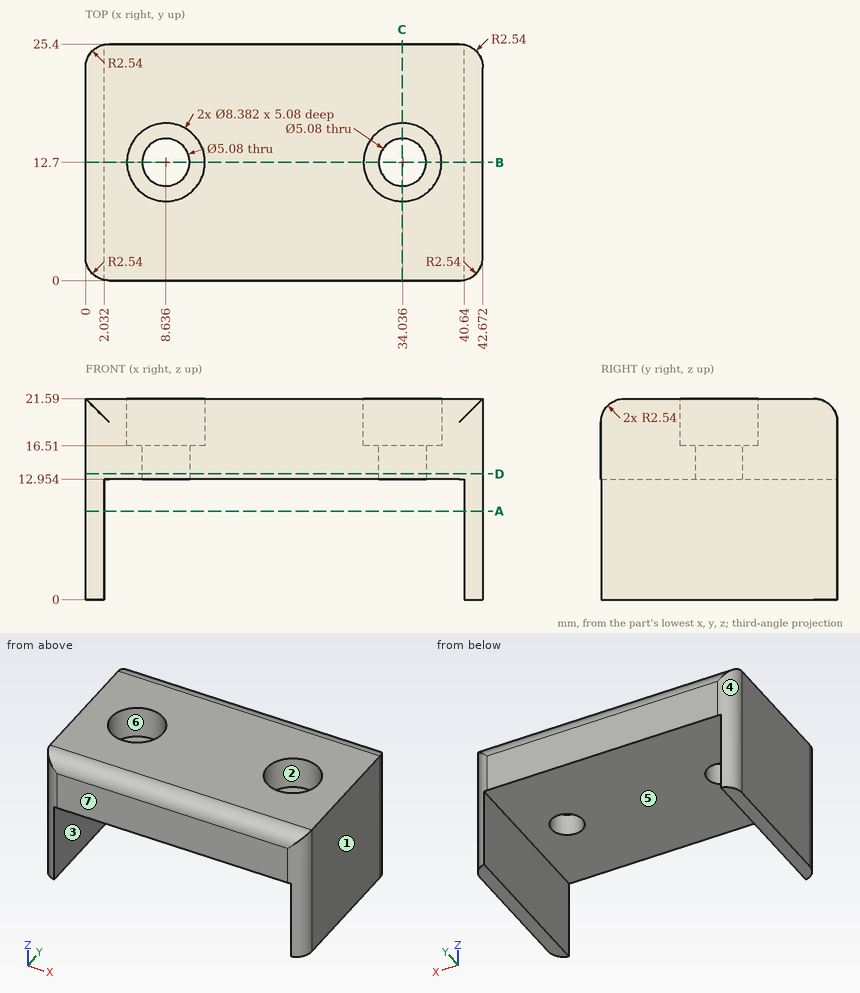
Here's the drawing with two shaded views (mm, measured from the low corner). I have some questions. A direction names the side the tool comes from. Give positions to 0.01 mm unless a question says otherwise; leave off trailing zeros. Loops run counter-clockwise (first coordinate to the right, second up) from the corner with the lowest first, then second, coordinate; pieces in that order, holes last. Notation, with made-up numbers: M 35,-10 L 88,-10 A20 ccw 88,14 Z; hole C 36.25,-25.75 d9. An arc over 180 degrees is marked long. One line per item, written item: value.
1) Imagine slicing it at B-B on y = 12.7. Write out the boundary of the cut face in (x, z) (3 decimals).
Geometry check:
outline: M 0,0 L 2.032,0 L 2.032,12.954 L 6.096,12.954 L 6.096,16.51 L 4.445,16.51 L 4.445,21.59 L 0,21.59 Z; M 11.176,12.954 L 31.496,12.954 L 31.496,16.51 L 29.845,16.51 L 29.845,21.59 L 12.827,21.59 L 12.827,16.51 L 11.176,16.51 Z; M 36.576,12.954 L 40.64,12.954 L 40.64,0 L 42.672,0 L 42.672,21.59 L 38.227,21.59 L 38.227,16.51 L 36.576,16.51 Z
2) On a 3-axis mill with a long thin cutter (end or side, diameter ignored), from which of +Z, -Z, +X, -X, +Y, -Y can I reach the whole of each face in a straight line? I mean the marked faces 5, 6 and 7. Say none if no direction works.
Geometry check:
face 5: -Z, +Y, -Y
face 6: +Z
face 7: +Z, -Z, +X, -X, -Y
3) Please list where these lines run through material, in increasing order: line 1 (X direction, y = 9.25, z = 7.25); line 2 (Z direction, x = 20.5, y = 3.75); line 3 (Z direction, x = 9.5, y = 10).
Geometry check:
line 1: x = 0 to 2.03, 40.64 to 42.67
line 2: z = 12.95 to 21.59
line 3: z = 12.95 to 16.51
4) I'm going to push flat-ended pins straight in: pin 1 (10 mm diameter, centred on y = 19.5, z = 7, fed in from -X); pin 2 (8 mm diameter, centred on x = 34.036, y = 12.7, fed in from +Z); pin 3 (10 mm diameter, centred on x = 19, y = 14.5, fed in from -Z); pin 4 (4.5 mm diameter, centred on x = 8.636, y = 12.7, fed in from +Z). Where does each tip first touch, or does it pass through?
Geometry check:
pin 1: stops at x = 0
pin 2: stops at z = 16.51
pin 3: stops at z = 12.95
pin 4: passes through
5) Thinking about a two-plate mould opening in X: for the marked faces 1, 2, 3 and 4, which applies, +X half, -X half, draft (parallel to the pull), parting line (faces both ways), or undercut?
Geometry check:
face 1: +X half
face 2: undercut
face 3: undercut
face 4: -X half
6) Imagine slicing it at A-A on z = 9.5. Write out the boundary of the cut face in (x, y), and give its area (3 significant figures).
Geometry check:
outline: M 0,2.54 A2.54 ccw 2.03,0.05 L 2.03,25.35 A2.54 ccw 0,22.86 Z; M 40.64,0.05 A2.54 ccw 42.67,2.54 L 42.67,22.86 A2.54 ccw 40.64,25.35 Z
area: 97.7 mm²
7) Imagine slicing it at C-C on x = 34. Write out the boundary of the cut face in (y, z).
Geometry check:
outline: M 0,12.95 L 10.16,12.95 L 10.16,16.51 L 8.51,16.51 L 8.51,21.59 L 2.54,21.59 A2.54 ccw 0,19.05 Z; M 15.24,12.95 L 25.4,12.95 L 25.4,19.05 A2.54 ccw 22.86,21.59 L 16.89,21.59 L 16.89,16.51 L 15.24,16.51 Z
8) Imagine slicing it at D-D on z = 13.5. Write out the boundary of the cut face in (x, y), and give its area (3 significant figures).
Geometry check:
outline: M 0,2.54 A2.54 ccw 2.54,0 L 40.13,0 A2.54 ccw 42.67,2.54 L 42.67,22.86 A2.54 ccw 40.13,25.4 L 2.54,25.4 A2.54 ccw 0,22.86 Z; hole C 8.64,12.7 d5.08; hole C 34.04,12.7 d5.08
area: 1,040 mm²
